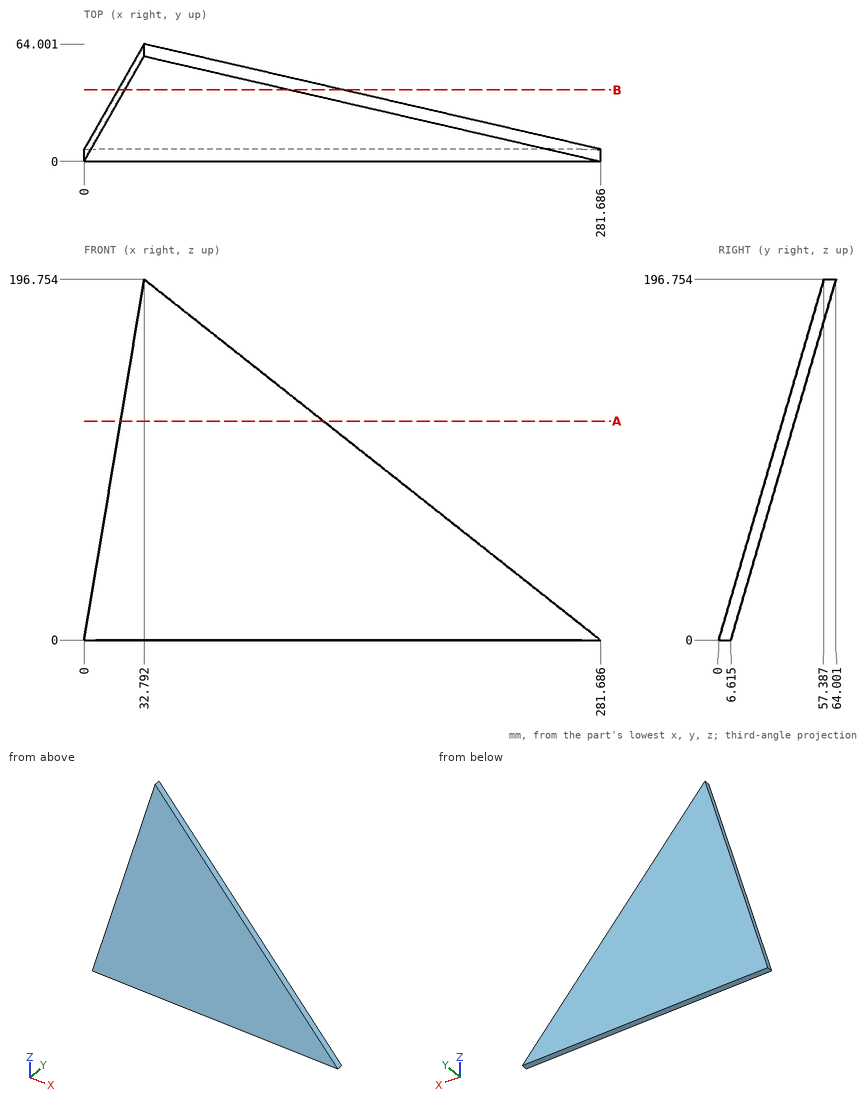
Geometry check sheet. Reference: drawing and pictorial views, mm from the part's lowest x, y, z. Coordinates: 2 decimals unless noted, no trailing zeros. Write each loop counter-clockwise with the first axis right and the second up, starting at its lowest first coordinate (ties: lowest second). Pieces come first, ordered by that corner, then holes. Notation, with made-up numbers: M 6,-38 L 20,-38 A16 ccw 20,-32 Z; hole C -39.5,44.5 d11. An arc over 180 degrees is marked long. Use one line per item in the form item = value.
Item 1: Material ranges on L1, parallel to Y at x = 76.5, z = 98; L2, parallel to Y at x = 139, z = 61.5, recorded low to high. Write a range as from..to.
Answer below:
L1 = 28.58..35.2
L2 = 17.94..24.55
Item 2: Gauge pin test, flat ends, axial feed: pin 1 Ø10 at (x, y) = (154.5, 36.5) entering from +Z (1 decimal); pin 2 Ø10 at (x, z) = (126, 75.5) entering from +Y; pin 3 Ø1.5 at (x, z) = (47.5, 166.5) entering from +Y (1 decimal). Record the tip position at first contact, or that the pin passes through.
Answer below:
pin_1 = 104.5
pin_2 = 30.09
pin_3 = 55.4
Item 3: Sectioned sample at A-A, the plane z = 119.5. Record the cut outline in (x, y) (1 decimal).
Answer below:
outline = M 19.9,34.9 L 130.5,34.9 L 130.5,41.5 L 19.9,41.5 Z
Item 4: Sectioned sample at B-B, the plane y = 39. Record the cut outline in (x, z) (1 decimal).
Answer below:
outline = M 18.5,111 L 141.2,111 L 112.5,133.7 L 22.3,133.7 Z
